from build123d import *

# Parameters (mm, degrees)
SKETCH_1_W      = 45
SKETCH_1_H      = 19.6
EXTRUDE_1_DEPTH = 1.6
SKETCH_2_R      = 8
EXTRUDE_2_DEPTH = 12
FILLET_1_R      = 1


with BuildPart() as part:
    # 草图1 → 凸台-拉伸1 (new body)
    with BuildSketch(Plane.XY):
        with Locations((22.5, 9.8)):
            Rectangle(SKETCH_1_W, SKETCH_1_H)
    extrude(amount=EXTRUDE_1_DEPTH)

    # 草图2 → 凸台-拉伸2 (add)
    with BuildSketch(Plane.XY.offset(1.6)):
        with Locations(Location((8.5, 9.8, 0), (0, 0, 180))):
            Circle(SKETCH_2_R)
        with Locations(Location((36.5, 9.8, 0), (0, 0, 180))):
            Circle(SKETCH_2_R)
    extrude(amount=EXTRUDE_2_DEPTH)

    # 圆角1
    fillet_1_edges = [part.edges().sort_by_distance(p)[0] for p in [
        (16.5, 9.8, 13.6),
        (44.5, 9.8, 13.6),
    ]]
    fillet(fillet_1_edges, radius=FILLET_1_R)


solid = part.part
Geometry check sheet. Reference: the model listing, model coordinates, mm. A direction names the side the tool comes from. Round coordinates to 2 decimals unless told otherwise and drop trailing zeros. Loops run counter-clockwise (first coordinate to the right, second up) from the corner with the lowest first, then second, coordinate; pieces in that order, holes last.
Item 1: Cross-section at A-A on y = 9.8. Record the boundary of the cut face in (x, z).
Item 2: Gauge pin test, flat ends, axial feed: pin 1 (3 mm diameter, centred on x = 34.5, y = 11.5, fed in from -Z); pin 2 (8 mm diameter, centred on y = 6, z = 10, fed in from -X); pin 3 (1 mm diameter, centred on x = 28.5, y = 14.5, fed in from +Z); pin 4 (1 mm diameter, centred on x = 9, y = 2, fed in from +Z). Record the tip position at first contact, or that the pin passes through.
Item 3: Cross-section at B-B on z = 8. Record the boundary of the cut face in (x, y).
Item 4: Thickness scan on line 1 (Z direction, x = 24, y = 1.75); line 2 (X direction, y = 8.75, z = 6.75); line 3 (X direction, y = 7.5, z = 9.75). Record the ranges inside material, lowest first.
Item 5: Cross-section at D-D on x = 28. Record the boundary of the cut face in (y, z), then the cut area to 3 significant figures.
Item 6: Access from +Z, -Z, +X, -X, +Y, -Y to the whole of each face (thin tool, end or side, straight path). Record for faces 1 (the cylindrical face through (14.4, 4.4, 7)), 2 (the flat face through (37, 10, 13.6)).
Item 7: Cross-section at C-C on x = 36.5. Record the boundary of the cut face in (y, z), then the cut area to 3 significant figures.
Item 8: Mould release check, pull along X, two halves, no side actions. Record for faces 3 (the flat face through (45, 10, 1)), 4 (the flat face through (0, 10, 1)), 5 (the flat face through (22, 19.6, 1)), 6 (the flat face through (22, 10, 1.6)): pulls with the +X half, pulls with the -X half, needs draft (parallel to the pull), parting line crosses it, or undercut.
Answer sheet:
1. outline: (0, 0) - (45, 0) - (45, 1.6) - (44.5, 1.6) - (44.5, 12.6) arc R1 ccw to (43.5, 13.6) - (29.5, 13.6) arc R1 ccw to (28.5, 12.6) - (28.5, 1.6) - (16.5, 1.6) - (16.5, 12.6) arc R1 ccw to (15.5, 13.6) - (1.5, 13.6) arc R1 ccw to (0.5, 12.6) - (0.5, 1.6) - (0, 1.6) - close
2. pin 1: stops at z = 0
2. pin 2: stops at x = 0.5
2. pin 3: stops at z = 1.6
2. pin 4: stops at z = 13.55
3. outline: circle Ø16 at (8.5, 9.8); circle Ø16 at (36.5, 9.8)
4. line 1: z = 0 to 1.6
4. line 2: x = 0.57 to 16.43, 28.57 to 44.43
4. line 3: x = 0.84 to 16.16, 28.84 to 44.16
5. outline: (0, 0) - (19.6, 0) - (19.6, 1.6) - (0, 1.6) - close
5. area: 31.4 mm2
6. face 1: +Z
6. face 2: +Z, +X, -X, +Y, -Y
7. outline: (0, 0) - (19.6, 0) - (19.6, 1.6) - (17.8, 1.6) - (17.8, 12.6) arc R1 ccw to (16.8, 13.6) - (2.8, 13.6) arc R1 ccw to (1.8, 12.6) - (1.8, 1.6) - (0, 1.6) - close
7. area: 223 mm2
8. face 3: pulls with the +X half
8. face 4: pulls with the -X half
8. face 5: needs draft
8. face 6: undercut
